```python
from build123d import *

# Parameters (mm, degrees)
F0_R     = 14.224
F0_R_2   = 9.5504
F1_DEPTH = 19.05
F2_R     = 14.224
F2_R_2   = 12.6365
F3_DEPTH = 1.5875
F4_SIZE  = 0.762


with BuildPart() as f1:
    # F0 (on Front) → F1 (new body, symmetric)
    with BuildSketch(Plane.XZ):
        Circle(F0_R)
        Circle(F0_R_2, mode=Mode.SUBTRACT)
    extrude(amount=F1_DEPTH, both=True)

    # F2 (on Front) → F3 (cut, symmetric)
    with BuildSketch(Plane.XZ):
        Circle(F2_R)
        Circle(F2_R_2, mode=Mode.SUBTRACT)
    extrude(amount=F3_DEPTH, both=True, mode=Mode.SUBTRACT)

    # F4
    f4_edges = [f1.edges().sort_by_distance(p)[0] for p in [
        (-14.224, 19.05, 0),
        (-14.224, -19.05, 0),
        (-9.5504, 19.05, 0),
        (-9.5504, -19.05, 0),
    ]]
    chamfer(f4_edges, length=F4_SIZE)


solid = f1.part
```
The listing builds one solid part. Answer for the finished solid, in the listing's coordinates (mm). A direction names the side the tool comes from. Give positions to 0.01 mm unless a question says otherwise; leave off trailing zeros. Loops run counter-clockwise (first coordinate to the right, second up) from the corner with the lowest first, then second, coordinate; pieces in that order, holes last. Notation, with made-up numbers: (-23, 50) - (18, 50) arc R25 cw to (18, 87) - close; hole circle Ø8 at (64.25, 2). An arc over 180 degrees is marked (long way). Answer as CSV lines item,"result". Start each with the question number.
Item 1: A cutting plane is placed at A-A on x = 0. Determine the outline of the cut face in (y, z), then the cut area to 3 significant figures.
Item 2: Find the intervals of material crossed by line 1 (Y direction, x = -9.5, z = 9.25); line 2 (Z direction, x = 0, y = -1); line 3 (Z direction, x = 0, y = -9.5), in increasing order. Write a range as from..to.
Item 3: A cutting plane is placed at B-B on z = 0. Determine the outline of the cut face in (x, y), then the cut area to 3 significant figures.
Item 4: Each of these flat-tipped pins is pushed along its axis until it touches: pin 1 (1 mm diameter, centred on x = 10, y = -10, fed in from -Z); pin 2 (1 mm diameter, centred on y = -0.5, z = 1.5, fed in from +X); pin 3 (6 mm diameter, centred on x = -6.5, z = 3, fed in from -Y). Where does it stop, or does it pass through?
Item 5: A cutting plane is placed at C-C on y = -16. Determine the outline of the cut face in (x, z), then the cut area to 3 significant figures.
Item 6: For faces 1 (the face through (0, 1.588, 13)), 2 (the face through (-3.083, 9.821, -13.886)), determine the directions among +Z, -Z, +X, -X, +Y, -Y from which every point of the face is accessible in a straight line to the end or side of a thin tool.
Item 7: The mould has two halves that part along X. Classify faces 3 (the face through (-2.07, 0.256, -9.323)), 4 (the face through (-3.083, -10.055, -13.886)), 5 (the face through (0, -1.588, 13)): +X half, -X half, draft (parallel to the pull), parting line (faces both ways), or undercut.
Found:
1,outline,"(-19.05, -13.46) - (-18.29, -14.22) - (-1.59, -14.22) - (-1.59, -12.64) - (1.59, -12.64) - (1.59, -14.22) - (18.29, -14.22) - (19.05, -13.46) - (19.05, -10.31) - (18.29, -9.55) - (-18.29, -9.55) - (-19.05, -10.31) - close; (-19.05, 10.31) - (-18.29, 9.55) - (18.29, 9.55) - (19.05, 10.31) - (19.05, 13.46) - (18.29, 14.22) - (1.59, 14.22) - (1.59, 12.64) - (-1.59, 12.64) - (-1.59, 14.22) - (-18.29, 14.22) - (-19.05, 13.46) - close"
1,area,"344 mm^2"
2,line 1,"y = -19.05..-1.59, 1.59..19.05"
2,line 2,"z = -12.64..-9.55, 9.55..12.64"
2,line 3,"z = -14.22..-9.55, 9.55..14.22"
3,outline,"(-14.22, -18.29) - (-13.46, -19.05) - (-10.31, -19.05) - (-9.55, -18.29) - (-9.55, 18.29) - (-10.31, 19.05) - (-13.46, 19.05) - (-14.22, 18.29) - (-14.22, 1.59) - (-12.64, 1.59) - (-12.64, -1.59) - (-14.22, -1.59) - close; (9.55, -18.29) - (10.31, -19.05) - (13.46, -19.05) - (14.22, -18.29) - (14.22, -1.59) - (12.64, -1.59) - (12.64, 1.59) - (14.22, 1.59) - (14.22, 18.29) - (13.46, 19.05) - (10.31, 19.05) - (9.55, 18.29) - close"
3,area,"344 mm^2"
4,pin 1,"stops at z = -10.59"
4,pin 2,"stops at x = 12.6"
4,pin 3,"stops at y = -18.9"
5,outline,"circle Ø28.45 at (0, 0); hole circle Ø19.1 at (0, 0)"
5,area,"349 mm^2"
6,face 1,"none"
6,face 2,"+Y, -Y"
7,face 3,"undercut"
7,face 4,"parting line"
7,face 5,"draft"
